Here's how the part is built. I have some questions about the finished solid (model axes, mm). Face numbers are marked on the shaded views. A direction names the side the tool comes from. Round coordinates to 2 decimals unless told otherwise and drop trailing zeros. Order: outer loops, then holes, each group sorted by start corner. A loop starts at its lowest first (then second) coordinate and runs counter-clockwise, first axis right, second up. Notation, with made-up numbers: (33, 54.5) -> (91, 54.5) arc R17 ccw to (91, 63.5) -> close; hole circle Ø1 at (62, 21). An arc over 180 degrees is marked (long way). Use a Markdown table: item, result. Add a question column.
(1) I want a section at A-A, the plane z = 17.5. Please give me the cut outline in (x, y).
(2) On a 3-axis mill with a long thin cutter (end or side, diameter ignored), from which of +Z, -Z, +X, -X, +Y, -Y can I reach the whole of each face in a straight line? I mean the marked faces 1 and 2. Say none if no direction works.
(3) Thinking about a two-plate mould opening in Y: for the marked faces 3, 4 and 5, which applies, pulls with the +Y half, pulls with the -Y half, needs draft (parallel to the pull), parting line crosses it, or undercut?
(4) I want a section at B-B, the plane y = 36. Please give me the cut outline in (x, z).
(5) If I drill on probe 1 along Y at (x, z) = (-6, 7.25); probe 2 along Z at (x, y) = (-39.5, -12); probe 3 along Z at (x, y) = (41, -21.5), over which ranges is the centre line in solid material (lowest first)?
(6) I'm going to push flat-ended pins straight in: P1, Ø8, axis at y = 19.5, z = 3.5, coming from the -X side; P2, Ø6, axis at y = 19.5, z = 3, coming from the +X side; P3, Ø12, axis at x = -23.5, z = 9.5, coming from the -Y side; P4, Ø2.5, axis at x = -45.99, y = 0.83, coming from the -Z side. Where does each tip first touch, or does it pass through?
(7) I want a section at C-C, the plane z = 11.5. Please give me the cut outline in (x, y), then the cut area to 3 significant figures.
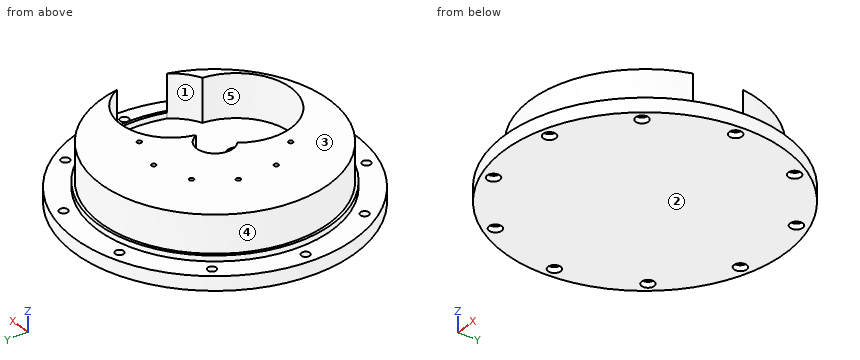
from build123d import *

# Parameters (mm, degrees)
SKETCH_1_R               = 50
EXTRUDE_1_DEPTH          = 5
EXTRUDE_START            = 5
SKETCH_1_10_R            = 41.75
SKETCH_1_10_R_2          = 40.75
EXTRUDE_2_DEPTH          = 2
SKETCH_1_8_R             = 1.5
CUT_EXTRUDE_1_DEPTH      = 72.056315694
SKETCH_1_9_R             = 2.25
CUT_EXTRUDE_2_DEPTH      = 2
PATTERN_CIRCULAR_1_COUNT = 10
EXTRUDE_3_DEPTH          = 15.3
SKETCH_3_R               = 0.8
CUT_EXTRUDE_3_DEPTH      = 4
PATTERN_CIRCULAR_2_COUNT = 10
SKETCH_4_R               = 3.1
CUT_EXTRUDE_4_DEPTH      = 2.6


with BuildPart() as part:
    # 草图1 → 凸台-拉伸1 (new body)
    with BuildSketch(Plane.XY):
        Circle(SKETCH_1_R)
    extrude(amount=EXTRUDE_1_DEPTH)

    # 草图1<10> → 凸台-拉伸2 (add)
    with BuildSketch(Plane.XY.offset(EXTRUDE_START)):
        Circle(SKETCH_1_10_R)
        Circle(SKETCH_1_10_R_2, mode=Mode.SUBTRACT)
    extrude(amount=EXTRUDE_2_DEPTH)

    # 草图1<8> → 切除-拉伸1 (cut, through all)
    with BuildSketch(Plane.XY):
        with Locations((-13.425009626, 43.997376246)):
            Circle(SKETCH_1_8_R)
    cut_extrude_1 = extrude(amount=CUT_EXTRUDE_1_DEPTH, mode=Mode.SUBTRACT)

    # 草图1<9> → 切除-拉伸2 (cut)
    with BuildSketch(Plane.XY):
        with Locations((-13.425009626, 43.997376246)):
            Circle(SKETCH_1_9_R)
    cut_extrude_2 = extrude(amount=CUT_EXTRUDE_2_DEPTH, mode=Mode.SUBTRACT)

    # 阵列(圆周)1: 切除-拉伸1, 切除-拉伸2 ×10 about axis
    pattern_circular_1_axis = Axis((0, 0, 0), (0, 0, 1))
    add([cut_extrude_1.rotate(pattern_circular_1_axis, i * 360 / PATTERN_CIRCULAR_1_COUNT) for i in range(1, PATTERN_CIRCULAR_1_COUNT)], mode=Mode.SUBTRACT)
    add([cut_extrude_2.rotate(pattern_circular_1_axis, i * 360 / PATTERN_CIRCULAR_1_COUNT) for i in range(1, PATTERN_CIRCULAR_1_COUNT)], mode=Mode.SUBTRACT)

    # 草图2 → 凸台-拉伸3 (add)
    with BuildSketch(Plane(origin=(0, 0, 5), x_dir=(-1, 0, 0), z_dir=(0, 0, -1))):
        with BuildLine():
            ThreePointArc((-6.017976905, 2.456410789), (3.82060414, 5.258610463), (4.195842623, -4.964363472))
            ThreePointArc((4.195842623, -4.964363472), (-4.96592188, -34.460078522), (-31.161250412, -18.09731903))
            ThreePointArc((-31.161250412, -18.09731903), (-35.692076103, -15.246050057), (-39.183964293, -11.188361914))
            ThreePointArc((-39.183964293, -11.188361914), (40.658588797, 2.72794007), (-40.327377462, 5.8536422))
            ThreePointArc((-40.327377462, 5.8536422), (-22.215964652, 16.310012331), (-6.440100033, 2.581172401))
            ThreePointArc((-6.440100033, 2.581172401), (-6.228686427, 2.519982708), (-6.017976905, 2.456410789))
        make_face()
    extrude(amount=-EXTRUDE_3_DEPTH)

    # 草图3 → 切除-拉伸3 (cut)
    with BuildSketch(Plane.XY.offset(20.3)):
        with Locations((0, 22)):
            Circle(SKETCH_3_R)
    cut_extrude_3 = extrude(amount=-CUT_EXTRUDE_3_DEPTH, mode=Mode.SUBTRACT)

    # 阵列(圆周)2: 切除-拉伸3 ×10 about axis
    pattern_circular_2_axis = Axis((0, 0, 0), (0, 0, 1))
    for i in range(1, PATTERN_CIRCULAR_2_COUNT):
        add(cut_extrude_3.rotate(pattern_circular_2_axis, i * 360 / PATTERN_CIRCULAR_2_COUNT), mode=Mode.SUBTRACT)

    # 草图4 → 切除-拉伸4 (cut)
    with BuildSketch(Plane.XY.offset(5)):
        with Locations((11.755705046, -16.180339888)):
            Circle(SKETCH_4_R)
    extrude(amount=-CUT_EXTRUDE_4_DEPTH, mode=Mode.SUBTRACT)


solid = part.part
Taken from the geometry:
| question | item | result |
|---|---|---|
| 1 | outline | (-4.2, -4.96) arc R6.5 cw (long way) to (6.02, 2.46) arc R19.5 cw to (6.44, 2.58) arc R18 cw to (40.33, 5.85) arc R40.75 ccw (long way) to (39.18, -11.19) arc R18 cw to (31.16, -18.1) arc R19.5 cw (long way) to start; hole circle Ø1.6 at (-20.92, -6.8); hole circle Ø1.6 at (-20.92, 6.8); hole circle Ø1.6 at (-12.93, -17.8); hole circle Ø1.6 at (-12.93, 17.8); hole circle Ø1.6 at (0, 22); hole circle Ø1.6 at (12.93, 17.8) |
| 2 | face 1 | +Z |
| 2 | face 2 | -Z, +X, -X, +Y, -Y |
| 3 | face 3 | needs draft |
| 3 | face 4 | parting line crosses it |
| 3 | face 5 | undercut |
| 4 | outline | (-34.7, 0) -> (34.7, 0) -> (34.7, 5) -> (21.14, 5) -> (21.14, 7) -> (19.09, 7) -> (19.09, 20.3) -> (-19.09, 20.3) -> (-19.09, 7) -> (-21.14, 7) -> (-21.14, 5) -> (-34.7, 5) -> close |
| 5 | probe 1 | y = -40.31 to -24.24, -8.12 to -2.5, 2.5 to 40.31 |
| 5 | probe 2 | z = 0 to 7 |
| 5 | probe 3 | z = 0 to 5 |
| 6 | P1 | stops at x = -47.54 |
| 6 | P2 | stops at x = 47.2 |
| 6 | P3 | stops at y = -46.03 |
| 6 | P4 | passes through |
| 7 | outline | (-4.2, -4.96) arc R6.5 cw (long way) to (6.02, 2.46) arc R19.5 cw to (6.44, 2.58) arc R18 cw to (40.33, 5.85) arc R40.75 ccw (long way) to (39.18, -11.19) arc R18 cw to (31.16, -18.1) arc R19.5 cw (long way) to start |
| 7 | area | 3,360 mm2 |
